Input: part model. Units: mm. Frame: model coordinates. Give positions to 0.01 mm unless a question says otherwise; leave off trailing zeros. Loops run counter-clockwise (first coordinate to the right, second up) from the corner with the lowest first, then second, coordinate; pieces in that order, holes last. Notation, with made-up numbers: M 45.25,-11 L 89.25,-11 A5 cw 89.25,-7 Z; hole C 52,35.25 d7. An arc over 180 degrees is marked long. Use a Markdown table: item, result. Add a question column.
from build123d import *

# Parameters (mm, degrees)
F0_W     = 25.4
F0_H     = 25.4
F1_DEPTH = 2.54
F3_DEPTH = 4.191
F4_DEPTH = 4.191
F7_DEPTH = 1.905


with BuildPart() as f1:
    # F0 (on Top) → F1 (new body)
    with BuildSketch(Plane.XY):
        with Locations((-37.877972, 34.147903)):
            Rectangle(F0_W, F0_H)
    extrude(amount=F1_DEPTH)

    # F2 (on face) → F3 (join)
    with BuildSketch(Plane.XY.offset(2.54)):
        Polygon((-38.830472, 24.622903), (-38.830472, 24.036821), (-38.830472, 23.352903), (-37.877972, 23.352903), (-36.925472, 23.352903), (-36.925472, 24.622903), align=None)
    extrude(amount=F3_DEPTH)

    # F2 (on face) → F4 (join)
    with BuildSketch(Plane.XY.offset(2.54)):
        Polygon((-36.925472, 44.942903), (-37.877972, 44.942903), (-38.830472, 44.942903), (-38.830472, 44.307903), (-38.830472, 43.672903), (-36.925472, 43.672903), align=None)
    extrude(amount=F4_DEPTH)

    # F6 (on face) + F5 (on face) → F7 (join)
    with BuildSketch(Plane(origin=(-38.830472, 0, 0), x_dir=(0, -1, 0), z_dir=(-1, 0, 0))):
        Polygon((-23.352903, 6.731), (-23.352903, 5.1435), (-22.590903, 5.1435), align=None)
    with BuildSketch(Plane(origin=(-38.830472, 0, 0), x_dir=(0, -1, 0), z_dir=(-1, 0, 0))):
        Polygon((-45.728009, 5.272041), (-44.942903, 5.272041), (-44.942903, 6.731), align=None)
    extrude(amount=-F7_DEPTH)


solid = f1.part
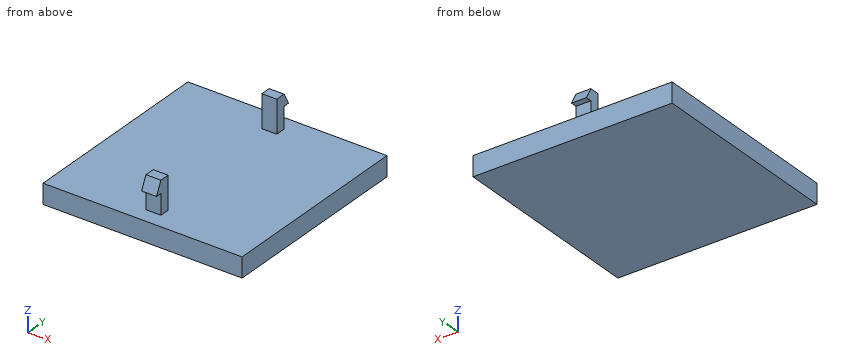
1) Contact query for flat-ended pins moving along their axis: P1, Ø2, axis at y = 24, z = 5.5, coming from the +X side; P2, Ø8, axis at x = -39, y = 35.5, coming from the +Z side; P3, Ø1.5, axis at x = -37.5, z = 4, coming from the -Y side. Output: stop coordinate, or through.
2) Section query C-C, the plane y = 38.75. Return the cut outline in (x, z).
3) Section query A-A, the plane z = 4.5. Return the cut outline in (x, y), and give its area (3 significant figures).
4) Section query B-B, the plane x = -42. Return the cut outline in (y, z).
5) Ray query, line 1 (Z direction, x = -36, y = 34.5); line 2 (X direction, y = 23.75, z = 3.5). Return the intervals inside material, ascending. Write a range as [from, to].
Entries:
| question | item | result |
|---|---|---|
| 1 | P1 | stops at x = -36.93 |
| 1 | P2 | stops at z = 2.54 |
| 1 | P3 | stops at y = 23.35 |
| 2 | outline | M -50.58,0 L -25.18,0 L -25.18,2.54 L -50.58,2.54 Z |
| 3 | outline | M -38.83,23.35 L -36.93,23.35 L -36.93,24.62 L -38.83,24.62 Z; M -38.83,43.67 L -36.93,43.67 L -36.93,44.94 L -38.83,44.94 Z |
| 3 | area | 4.84 mm² |
| 4 | outline | M 21.45,0 L 46.85,0 L 46.85,2.54 L 21.45,2.54 Z |
| 5 | line 1 | z = [0, 2.54] |
| 5 | line 2 | x = [-38.83, -36.93] |
